Could you check a few things on this model? Use its own coordinates, in mm. A direction names the side the tool comes from. Give positions to 0.01 mm unless a question says otherwise; leave off trailing zeros. Order: outer loops, then holes, each group sorted by start corner. A loop starts at its lowest first (then second) coordinate and runs counter-clockwise, first axis right, second up. Notation, with made-up numbers: M -31,22.25 L 5,22.25 A16 ccw 5,52.25 Z; hole C 54.5,23.25 d2. An arc over 180 degrees is marked long. Use a Markdown table: item, result. Add a question column.
Autodesk Inventor part; units mm, degrees
ref_plane "YZ Plane" through (0, 0, 0) normal (1, 0, 0) x (0, 1, 0)
ref_plane "XZ Plane" through (0, 0, 0) normal (0, 1, 0) x (-1, 0, 0)
ref_plane "XY Plane" through (0, 0, 0) normal (0, 0, 1) x (1, 0, 0)
sketch "草圖2" plane through (0, 0, 0) normal (0, 1, 0) x (-1, 0, 0)
  line L0 (0, 0) -> (31, 0)
  line L1 (31, 0) -> (31, -14)
  line L2 (31, -14) -> (0, -14)
  line L3 (0, -14) -> (0, 0)
  line L4 (31, -14) -> (28, -14)
  line L5 (28, -14) -> (28, -17)
  line L6 (28, -17) -> (31, -17)
  line L7 (31, -17) -> (31, -14)
  line L8 (31, -7) -> (0, -7)
  line L9 (15.5, -14) -> (15.5, 0)
  line L10 (28, 0) -> (28, 3)
  line L11 (28, 3) -> (31, 3)
  line L12 (31, 3) -> (31, 0)
  line L13 (3, -14) -> (3, -17)
  line L14 (3, -17) -> (0, -17)
  line L15 (0, -17) -> (0, -14)
  line L16 (3, 0) -> (3, 3)
  line L17 (3, 3) -> (0, 3)
  line L18 (0, 3) -> (0, 0)
  line L19 (17, -14) -> (14, -14)
  line L20 (14, -14) -> (14, -17)
  line L21 (14, -17) -> (17, -17)
  line L22 (17, -17) -> (17, -14)
  line L23 (14, 0) -> (14, 3)
  line L24 (14, 3) -> (17, 3)
  line L25 (17, 3) -> (17, 0)
  line L26 (31, 0) -> (46, 0)
  line L27 (46, 0) -> (46, -14)
  line L28 (46, -14) -> (31, -14)
  line L29 (31, -14) -> (31, 0)
  line L30 (45, -14) -> (42, -14)
  line L31 (42, -14) -> (42, -17)
  line L32 (42, 0) -> (42, 3)
  line L33 (42, -17) -> (46, -17)
  line L34 (46, -14) -> (46, -17)
  line L35 (42, 3) -> (46, 3)
  line L36 (46, 0) -> (46, 3)
  point P0 (44, 3)
  dimension "d9" = 31
  dimension "d10" = 14
  dimension "d11" = 3
  dimension "d12" = 3
  dimension "d13" = 3
  dimension "d14" = 3
  dimension "d18" = 11
  dimension "d21" = 14
  dimension "d22" = 46
  dimension "d23" = 20
extrude "擠出2" add sketch "草圖2" along normal blind 3
properties material "MDF Medium Density Fiberboard"
1) Suppose I cut it at A-A on z = -15.25. Please give me the cut outline in (x, y), and give its area (3 significant figures).
2) Please list where these lines run through material, in increasing order: line 1 (X direction, y = 0.1, z = -15); line 2 (Z direction, x = -40, y = 2.35). Write a range as from..to.
3) Suppose I cut it at B-B on y = 1.2. Please give me the cut outline in (x, z).
4) For faces 4 (the face through (-28, 1, 1)), 5 (the face through (-15, 1, -17)), 6 (the face through (-17, 1, -16)), which set-ups out of +Z, -Z, +X, -X, +Y, -Y let a thin tool reach every point of the face, with its end or its side?
5) For pin 1 (1.5 mm diameter, centred on x = -21, y = 2, fed in from -Z); pin 2 (1.5 mm diameter, centred on x = -8.5, y = 1.5, fed in from +Z), each with a flat end and sliding along its axis, tell me the tip position at first contact or that it passes through.
6) We'd pull the mould along X, two halves only. Please class faces 1 (the face through (-2, 1, -17)), 2 (the face through (0, 1, -7)), 3 (the face through (-22, 1, 0)): pulls with the +X half, pulls with the -X half, needs draft (parallel to the pull), parting line crosses it, or undercut.
7) Suppose I cut it at C-C on x = -35.5. Please give me the cut outline in (y, z).
Values found:
| question | item | result |
|---|---|---|
| 1 | outline | M -46,0 L -42,0 L -42,3 L -46,3 Z; M -31,0 L -28,0 L -28,3 L -31,3 Z; M -17,0 L -14,0 L -14,3 L -17,3 Z; M -3,0 L 0,0 L 0,3 L -3,3 Z |
| 1 | area | 39.0 mm^2 |
| 2 | line 1 | x = -46..-42, -31..-28, -17..-14, -3..0 |
| 2 | line 2 | z = -14..0 |
| 3 | outline | M -46,-17 L -42,-17 L -42,-14 L -31,-14 L -31,-17 L -28,-17 L -28,-14 L -17,-14 L -17,-17 L -14,-17 L -14,-14 L -3,-14 L -3,-17 L 0,-17 L 0,3 L -3,3 L -3,0 L -14,0 L -14,3 L -17,3 L -17,0 L -28,0 L -28,3 L -31,3 L -31,0 L -42,0 L -42,3 L -46,3 Z |
| 4 | face 4 | +Z, +Y, -Y |
| 4 | face 5 | -Z, +X, -X, +Y, -Y |
| 4 | face 6 | -Z, +Y, -Y |
| 5 | pin 1 | stops at z = -14 |
| 5 | pin 2 | stops at z = 0 |
| 6 | face 1 | needs draft |
| 6 | face 2 | pulls with the +X half |
| 6 | face 3 | undercut |
| 7 | outline | M 0,-14 L 3,-14 L 3,0 L 0,0 Z |
